```python
from build123d import *

# Parameters (mm, degrees)
SKETCH1_W           = 73.5
SKETCH1_H           = 37.5
SKETCH1_R           = 1.25
SKETCH1_W_2         = 53.3
SKETCH1_H_2         = 32.1
SKETCH1_W_3         = 2.5
SKETCH1_H_3         = 15
BOSS_EXTRUDE1_DEPTH = 6.18


with BuildPart() as part:
    # Sketch1 → Boss-Extrude1 (new body)
    with BuildSketch(Plane(origin=(0, 0, 0), x_dir=(1, 0, 0), z_dir=(0, 1, 0))):
        with Locations((36.75, -18.75)):
            Rectangle(SKETCH1_W, SKETCH1_H)
        with Locations(Location((2.3, -34.5, 0), (0, 0, 270))):
            Circle(SKETCH1_R, mode=Mode.SUBTRACT)
        with Locations(Location((2.3, -3, 0), (0, 0, 270))):
            Circle(SKETCH1_R, mode=Mode.SUBTRACT)
        with Locations((38.65, -18.75)):
            Rectangle(SKETCH1_W_2, SKETCH1_H_2, mode=Mode.SUBTRACT)
        with Locations(Location((71.2, -3, 0), (0, 0, 270))):
            Circle(SKETCH1_R, mode=Mode.SUBTRACT)
        with Locations(Location((71.2, -34.5, 0), (0, 0, 270))):
            Circle(SKETCH1_R, mode=Mode.SUBTRACT)
        with Locations((70.5, -19.5)):
            Rectangle(SKETCH1_W_3, SKETCH1_H_3, mode=Mode.SUBTRACT)
    extrude(amount=BOSS_EXTRUDE1_DEPTH)


solid = part.part
```
Geometry: final body of the model. Coordinates: model frame, mm. A direction names the side the tool comes from. Give positions to 0.01 mm unless a question says otherwise; leave off trailing zeros. Write each loop counter-clockwise with the first axis right and the second up, starting at its lowest first coordinate (ties: lowest second). Pieces come first, ordered by that corner, then holes.
1. Section query A-A, the plane z = 14.5. Return loops of the section in (x, y), then the cut area to 3 significant figures.
2. Section query C-C, the plane x = 23. Return loops of the section in (y, z), then the cut area to 3 significant figures.
3. Draft query along X for faces 1 (the flat face through (0, 3, 19)), 2 (the flat face through (28, 0, 35)), 3 (the flat face through (12, 3, 19)). Return one class per face: released by +X, released by -X, zero draft, split by the parting line, or undercut.
4. Section query D-D, the plane z = 9. Return loops of the section in (x, y).
5. Reachability of faces 4 (the flat face through (28, 6.18, 35)), 5 (the flat face through (70, 3, 27)) from +Z, -Z, +X, -X, +Y, -Y: full face, straight path, thin tool, end or side. Return the list, or none.
6. Line query: probe 1 along Z at (x, y) = (71.2, 1.5); probe 2 along X at (y, z) = (2.75, 3); probe 3 along X at (y, z) = (3.25, 16.5). Output: solid intervals per line, ascending.
7. Section query B-B, the plane y = 2.75. Return loops of the section in (x, z), then the cut area to 3 significant figures.
Computed:
1. outline: (0, 0) - (12, 0) - (12, 6.18) - (0, 6.18) - close; (65.3, 0) - (69.25, 0) - (69.25, 6.18) - (65.3, 6.18) - close; (71.75, 0) - (73.5, 0) - (73.5, 6.18) - (71.75, 6.18) - close
1. area: 109 mm2
2. outline: (0, 0) - (6.18, 0) - (6.18, 2.7) - (0, 2.7) - close; (0, 34.8) - (6.18, 34.8) - (6.18, 37.5) - (0, 37.5) - close
2. area: 33.4 mm2
3. face 1: released by -X
3. face 2: zero draft
3. face 3: undercut
4. outline: (0, 0) - (12, 0) - (12, 6.18) - (0, 6.18) - close; (65.3, 0) - (73.5, 0) - (73.5, 6.18) - (65.3, 6.18) - close
5. face 4: +Z, -Z, +X, -X, +Y
5. face 5: +Y, -Y
6. probe 1: z = 0 to 1.75, 4.25 to 12, 27 to 33.25, 35.75 to 37.5
6. probe 2: x = 0 to 1.05, 3.55 to 12, 65.3 to 69.95, 72.45 to 73.5
6. probe 3: x = 0 to 12, 65.3 to 69.25, 71.75 to 73.5
7. outline: (0, 0) - (73.5, 0) - (73.5, 37.5) - (0, 37.5) - close; hole circle Ø2.5 at (2.3, 3); hole circle Ø2.5 at (2.3, 34.5); hole (12, 2.7) - (65.3, 2.7) - (65.3, 34.8) - (12, 34.8) - close; hole (69.25, 12) - (71.75, 12) - (71.75, 27) - (69.25, 27) - close; hole circle Ø2.5 at (71.2, 3); hole circle Ø2.5 at (71.2, 34.5)
7. area: 988 mm2
